Check sheet for the modelled part. Datum: model origin and axes. Units: mm. A direction names the side the tool comes from. Coordinates: 2 decimals unless noted, no trailing zeros. Loops run counter-clockwise (first coordinate to the right, second up) from the corner with the lowest first, then second, coordinate; pieces in that order, holes last.
```python
from build123d import *

# Parameters (mm, degrees)
F0_R     = 7.95
F1_DEPTH = 3.1
F2_R     = 10
F3_DEPTH = 3.77
F4_R     = 7.95
F5_DEPTH = 3.22
F6_R     = 1.55
F7_DEPTH = 25
F8_R     = 7.5
F8_R_2   = 1.55
F8_R_3   = 2.925
F8_R_4   = 0.8
F9_DEPTH = 9


with BuildPart() as f1:
    # F0 (on Top) → F1 (new body)
    with BuildSketch(Plane.XY):
        with Locations((-16.1596555263, 42.1727597713)):
            Circle(F0_R)
    extrude(amount=F1_DEPTH)

    # F2 (on face) → F3 (join)
    with BuildSketch(Plane.XY.offset(3.1)):
        with Locations((-16.1596555263, 42.1727597713)):
            Circle(F2_R)
    extrude(amount=F3_DEPTH)

    # F4 (on face) → F5 (join)
    with BuildSketch(Plane.XY.offset(6.87)):
        with Locations((-16.1596555263, 42.1727597713)):
            Circle(F4_R)
    extrude(amount=F5_DEPTH)

    # F6 (on face) → F7 (cut)
    with BuildSketch(Plane.XY.offset(10.09)):
        with Locations((-15.7605068353, 47.6678920378)):
            Circle(F6_R)
        with Locations((-19.8955421826, 45.8926504552)):
            Circle(F6_R)
        with Locations((-21.4543696493, 41.3926504552)):
            Circle(F6_R)
        with Locations((-18.3753594756, 38.1109289024)):
            Circle(F6_R)
        with Locations((-13.8753594756, 37.7701377139)):
            Circle(F6_R)
        with Locations((-10.8317825943, 41.0847477615)):
            Circle(F6_R)
        with Locations((-11.7717087802, 45.5847477615)):
            Circle(F6_R)
    extrude(amount=-F7_DEPTH, mode=Mode.SUBTRACT)

    # F8 (on face) → F9 (cut)
    with BuildSketch(Plane(origin=(0, 0, 0), x_dir=(1, 0, 0), z_dir=(0, 0, -1))):
        with Locations((-16.1596555263, -42.1727597713)):
            Circle(F8_R)
        with Locations((-19.8955421826, -45.8926504552)):
            Circle(F8_R_2, mode=Mode.SUBTRACT)
        with Locations((-16.1596555263, -42.1727597713)):
            Circle(F8_R_3, mode=Mode.SUBTRACT)
        with Locations((-15.7605068353, -47.6678920378)):
            Circle(F8_R_2, mode=Mode.SUBTRACT)
        with Locations((-11.7717087802, -45.5847477615)):
            Circle(F8_R_2, mode=Mode.SUBTRACT)
        with Locations((-21.4543696493, -41.3926504552)):
            Circle(F8_R_2, mode=Mode.SUBTRACT)
        with Locations((-18.3753594756, -38.1109289024)):
            Circle(F8_R_2, mode=Mode.SUBTRACT)
        with Locations((-10.8317825943, -41.0847477615)):
            Circle(F8_R_2, mode=Mode.SUBTRACT)
        with Locations((-13.8753594756, -37.7701377139)):
            Circle(F8_R_2, mode=Mode.SUBTRACT)
        with Locations((-16.1596555263, -42.1727597713)):
            Circle(F8_R_4)
    extrude(amount=-F9_DEPTH, mode=Mode.SUBTRACT)


solid = f1.part
```
1) Section check C-C on z = 5.5. Enter the section's corners in (x, y) (3 decimals).
Answer sheet:
outline: circle Ø20 at (-16.16, 42.173); circle Ø5.85 at (-16.16, 42.173); hole circle Ø15 at (-16.16, 42.173); hole circle Ø1.6 at (-16.16, 42.173)
2) Scan lines: line 1 (X direction, y = 40.25, z = 1.5); line 2 (Y direction, x = -16.25, z = 5); line 3 (Y direction, x = -16, z = 7.25). Record each from-to range of solid material in increasing order.
Answer sheet:
line 1: x = -23.87 to -23.41, -18.36 to -13.96, -8.91 to -8.45
line 2: y = 32.17 to 34.67, 39.25 to 41.38, 42.97 to 45.1, 49.67 to 52.17
line 3: y = 34.22 to 34.67, 39.25 to 41.39, 42.96 to 45.09, 49.67 to 50.12
3) Depth check by flat-ended pin: pin 1 (3 mm diameter, centred on x = -21.45, y = 41.39, fed in from +Z); pin 2 (4 mm diameter, centred on x = -19.9, y = 45.89, fed in from -Z); pin 3 (1.5 mm diameter, centred on x = -23, y = 36.5, fed in from -Z); pin 4 (2 mm diameter, centred on y = 43.5, z = 8.5, fed in from -X). Enter the tip coordinate at first touch or a pass-through.
Answer sheet:
pin 1: passes through
pin 2: stops at z = 9
pin 3: stops at z = 3.1
pin 4: stops at x = -24.1
4) Section check A-A on x = -12. Enter the section's corners in (y, z), plus the area to 3 significant figures.
Answer sheet:
outline: (33.08, 3.1) - (35.4, 3.1) - (35.4, 0) - (35.93, 0) - (35.93, 9) - (40.07, 9) - (40.07, 10.09) - (35.4, 10.09) - (35.4, 6.87) - (33.08, 6.87) - close; (42.1, 9) - (44.05, 9) - (44.05, 10.09) - (42.1, 10.09) - close; (47.12, 9) - (48.41, 9) - (48.41, 0) - (48.95, 0) - (48.95, 3.1) - (51.27, 3.1) - (51.27, 6.87) - (48.95, 6.87) - (48.95, 10.09) - (47.12, 10.09) - close
area: 36.3 mm2
5) Mould release check, pull along Y, two halves, no side actions. Record for faces 1 (the cylindrical face through (-19.06, 47.2, 9.55)), 2 (the cylindrical face through (-17.461, 52.088, 4.959)), 3 (the flat face through (-17, 34, 6.87)), 4 (the cylindrical face through (-13, 44.64, 9.55)): +Y half, -Y half, draft (parallel to the pull), parting line (faces both ways), or undercut.
Answer sheet:
face 1: undercut
face 2: parting line
face 3: draft
face 4: undercut
6) Section check B-B on y = 41.75. Give the number of separate pieces and of enclosed holes in the cut face, plus the area to 3 significant figures.
Answer sheet:
separate pieces: 3
enclosed holes: 0
area: 74.4 mm2
7) Section check D-D on y = 35. Enter the section's corners in (x, z), plus the area to 3 significant figures.
Answer sheet:
outline: (-23.13, 3.1) - (-19.59, 3.1) - (-19.59, 0) - (-18.35, 0) - (-18.35, 9) - (-13.97, 9) - (-13.97, 0) - (-12.73, 0) - (-12.73, 3.1) - (-9.19, 3.1) - (-9.19, 6.87) - (-12.73, 6.87) - (-12.73, 10.09) - (-19.59, 10.09) - (-19.59, 6.87) - (-23.13, 6.87) - close
area: 56.4 mm2
8) Set-up check for faces 5 (the flat face through (-17, 34, 3.1)), 6 (the cylindrical face through (-16.9, 48.72, 9.55)), 7 (the cylindrical face through (-12.49, 35.12, 8.46)): record each of +Z, -Z, +X, -X, +Y, -Y from which the full face is reachable in a straight line by a thin tool's end or side.
Answer sheet:
face 5: -Z
face 6: +Z, -Z
face 7: +Z
